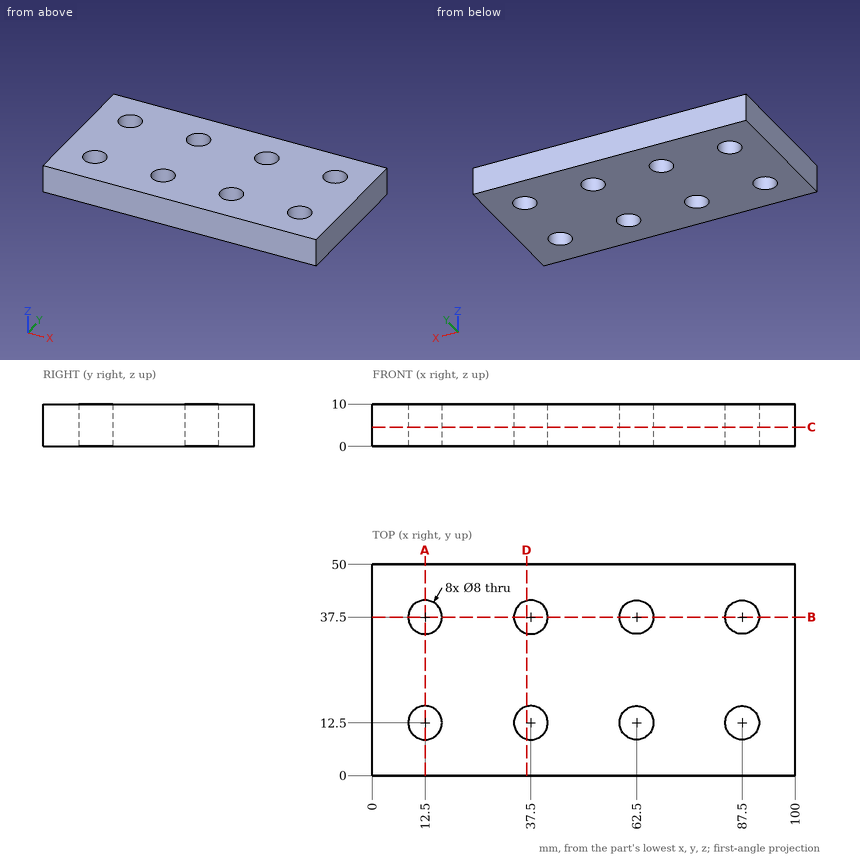
Source: three-view drawing plus pictorial views. Frame: mm from the lowest corner of the part. Give positions to 0.01 mm unless a question says otherwise; leave off trailing zeros. Order: outer loops, then holes, each group sorted by start corner. A loop starts at its lowest first (then second) coordinate and runs counter-clockwise, first axis right, second up. Notation, with made-up numbers: (39, -37.75) -> (91, -37.75) arc R24 ccw to (91, -4.75) -> close; hole circle Ø3 at (63.5, 8). An arc over 180 degrees is marked (long way). Put each result on its own line as item: value.
Q1. Section D-D, the plane x = 36.5. Return loops of the section in (y, z).
Here are the results:
outline: (0, 0) -> (8.63, 0) -> (8.63, 10) -> (0, 10) -> close; (16.37, 0) -> (33.63, 0) -> (33.63, 10) -> (16.37, 10) -> close; (41.37, 0) -> (50, 0) -> (50, 10) -> (41.37, 10) -> close
Q2. Section C-C, the plane z = 4.5. Count the separate pieces of the cut face and the enclosed holes in it, then the cut area to 3 significant figures.
Here are the results:
separate pieces: 1
enclosed holes: 8
area: 4,600 mm^2
Q3. Section A-A, the plane x = 12.5. Return loops of the section in (y, z), then the cut area to 3 significant figures.
Here are the results:
outline: (0, 0) -> (8.5, 0) -> (8.5, 10) -> (0, 10) -> close; (16.5, 0) -> (33.5, 0) -> (33.5, 10) -> (16.5, 10) -> close; (41.5, 0) -> (50, 0) -> (50, 10) -> (41.5, 10) -> close
area: 340 mm^2
Q4. Material intervals for L1, parallel to Y at x = 62.5, z = 4; L2, parallel to X at y = 10.5, z = 4.75; L3, parallel to X at y = 9, z = 5.75, sorted ascending.
Here are the results:
L1: y = 0 to 8.5, 16.5 to 33.5, 41.5 to 50
L2: x = 0 to 9.04, 15.96 to 34.04, 40.96 to 59.04, 65.96 to 84.04, 90.96 to 100
L3: x = 0 to 10.56, 14.44 to 35.56, 39.44 to 60.56, 64.44 to 85.56, 89.44 to 100
Q5. Section B-B, the plane y = 37.5. Return loops of the section in (x, z), then the cut area to 3 significant figures.
Here are the results:
outline: (0, 0) -> (8.5, 0) -> (8.5, 10) -> (0, 10) -> close; (16.5, 0) -> (33.5, 0) -> (33.5, 10) -> (16.5, 10) -> close; (41.5, 0) -> (58.5, 0) -> (58.5, 10) -> (41.5, 10) -> close; (66.5, 0) -> (83.5, 0) -> (83.5, 10) -> (66.5, 10) -> close; (91.5, 0) -> (100, 0) -> (100, 10) -> (91.5, 10) -> close
area: 680 mm^2
Q6. Pin query (flat end, axial travel): pin 1 (5 mm diameter, centred on x = 12.5, y = 37.5, fed in from +Z). Return the tip coordinate at first contact, or that it passes through.
Here are the results:
pin 1: passes through
